from build123d import *

# Parameters (mm, degrees)
F2_W     = 2.1
F2_H     = 15
F2_W_2   = 15
F2_H_2   = 2.1
F2_R     = 1.5
F2_W_3   = 43.75
F2_H_3   = 19.25
F3_DEPTH = 1.5
F4_DEPTH = 4.7
F5_DEPTH = 6
F6_R     = 1.5


with BuildPart() as f3:
    # F2 (on Top) → F3 (new body)
    with BuildSketch(Plane.XY):
        Polygon((-51.25, 18.5100111359), (-51.25, 26.75), (-43.0100111359, 26.75), (-7.5, 26.75), (-7.5, 28.85), (-53.35, 28.85), (-53.35, 7.5), (-51.25, 7.5), align=None)
        with Locations((-52.3, 0)):
            Rectangle(F2_W, F2_H)
        with Locations((52.3, 0)):
            Rectangle(F2_W, F2_H)
        Polygon((7.5, 28.85), (7.5, 26.75), (43.0100111359, 26.75), (51.25, 26.75), (51.25, 18.5100111359), (51.25, 7.5), (53.35, 7.5), (53.35, 28.85), align=None)
        Polygon((-51.25, -18.5100111359), (-51.25, -7.5), (-53.35, -7.5), (-53.35, -28.85), (-7.5, -28.85), (-7.5, -26.75), (-43.0100111359, -26.75), (-51.25, -26.75), align=None)
        with Locations((0, -27.8)):
            Rectangle(F2_W_2, F2_H_2)
        with Locations((0, 27.8)):
            Rectangle(F2_W_2, F2_H_2)
        Polygon((53.35, -7.5), (51.25, -7.5), (51.25, -18.5100111359), (51.25, -26.75), (43.0100111359, -26.75), (7.5, -26.75), (7.5, -28.85), (53.35, -28.85), align=None)
        with BuildLine():
            Line((-7.5, -7.5), (-51.25, -7.5))
            Line((-51.25, -7.5), (-51.25, -18.5100111359))
            ThreePointArc((-51.25, -18.5100111359), (-43.3634253301, -18.8634253301), (-43.0100111359, -26.75))
            Line((-43.0100111359, -26.75), (-7.5, -26.75))
            Line((-7.5, -26.75), (-7.5, -7.5))
        make_face()
        with BuildLine():
            Line((-43.0100111359, 26.75), (-51.25, 26.75))
            Line((-51.25, 26.75), (-51.25, 18.5100111359))
            ThreePointArc((-51.25, 18.5100111359), (-43.3634253301, 18.8634253301), (-43.0100111359, 26.75))
        make_face()
        with Locations((-47.5, 23)):
            Circle(F2_R, mode=Mode.SUBTRACT)
        with BuildLine():
            Line((51.25, 26.75), (43.0100111359, 26.75))
            ThreePointArc((43.0100111359, 26.75), (43.3634253301, 18.8634253301), (51.25, 18.5100111359))
            Line((51.25, 18.5100111359), (51.25, 26.75))
        make_face()
        with Locations((47.5, 23)):
            Circle(F2_R, mode=Mode.SUBTRACT)
        with BuildLine():
            Line((51.25, -26.75), (51.25, -18.5100111359))
            ThreePointArc((51.25, -18.5100111359), (43.3634253301, -18.8634253301), (43.0100111359, -26.75))
            Line((43.0100111359, -26.75), (51.25, -26.75))
        make_face()
        with Locations((47.5, -23)):
            Circle(F2_R, mode=Mode.SUBTRACT)
        with BuildLine():
            ThreePointArc((-43.0100111359, -26.75), (-43.3634253301, -18.8634253301), (-51.25, -18.5100111359))
            Line((-51.25, -18.5100111359), (-51.25, -26.75))
            Line((-51.25, -26.75), (-43.0100111359, -26.75))
        make_face()
        with Locations((-47.5, -23)):
            Circle(F2_R, mode=Mode.SUBTRACT)
        with Locations((-29.375, 0)):
            Rectangle(F2_W_3, F2_H)
        with Locations((-47.5, 0)):
            Circle(F2_R, mode=Mode.SUBTRACT)
        with BuildLine():
            Line((-7.5, 26.75), (-43.0100111359, 26.75))
            ThreePointArc((-43.0100111359, 26.75), (-43.3634253301, 18.8634253301), (-51.25, 18.5100111359))
            Line((-51.25, 18.5100111359), (-51.25, 7.5))
            Line((-51.25, 7.5), (-7.5, 7.5))
            Line((-7.5, 7.5), (-7.5, 26.75))
        make_face()
        with Locations((0, 17.125)):
            Rectangle(F2_W_2, F2_H_3)
        with Locations((0, 23)):
            Circle(F2_R, mode=Mode.SUBTRACT)
        with BuildLine():
            Line((43.0100111359, 26.75), (7.5, 26.75))
            Line((7.5, 26.75), (7.5, 7.5))
            Line((7.5, 7.5), (51.25, 7.5))
            Line((51.25, 7.5), (51.25, 18.5100111359))
            ThreePointArc((51.25, 18.5100111359), (43.3634253301, 18.8634253301), (43.0100111359, 26.75))
        make_face()
        with Locations((29.375, 0)):
            Rectangle(F2_W_3, F2_H)
        with Locations((47.5, 0)):
            Circle(F2_R, mode=Mode.SUBTRACT)
        with BuildLine():
            Line((51.25, -7.5), (7.5, -7.5))
            Line((7.5, -7.5), (7.5, -26.75))
            Line((7.5, -26.75), (43.0100111359, -26.75))
            ThreePointArc((43.0100111359, -26.75), (43.3634253301, -18.8634253301), (51.25, -18.5100111359))
            Line((51.25, -18.5100111359), (51.25, -7.5))
        make_face()
        with Locations((0, -17.125)):
            Rectangle(F2_W_2, F2_H_3)
        with Locations((0, -23)):
            Circle(F2_R, mode=Mode.SUBTRACT)
        Rectangle(F2_W_2, F2_H)
    extrude(amount=F3_DEPTH)

    # F2 (on Top) → F4 (join)
    with BuildSketch(Plane.XY):
        with BuildLine():
            ThreePointArc((-43.0100111359, -26.75), (-43.3634253301, -18.8634253301), (-51.25, -18.5100111359))
            Line((-51.25, -18.5100111359), (-51.25, -26.75))
            Line((-51.25, -26.75), (-43.0100111359, -26.75))
        make_face()
        with Locations((-47.5, -23)):
            Circle(F2_R, mode=Mode.SUBTRACT)
        with BuildLine():
            Line((51.25, -26.75), (51.25, -18.5100111359))
            ThreePointArc((51.25, -18.5100111359), (43.3634253301, -18.8634253301), (43.0100111359, -26.75))
            Line((43.0100111359, -26.75), (51.25, -26.75))
        make_face()
        with Locations((47.5, -23)):
            Circle(F2_R, mode=Mode.SUBTRACT)
        with BuildLine():
            Line((51.25, 26.75), (43.0100111359, 26.75))
            ThreePointArc((43.0100111359, 26.75), (43.3634253301, 18.8634253301), (51.25, 18.5100111359))
            Line((51.25, 18.5100111359), (51.25, 26.75))
        make_face()
        with Locations((47.5, 23)):
            Circle(F2_R, mode=Mode.SUBTRACT)
        with BuildLine():
            Line((-43.0100111359, 26.75), (-51.25, 26.75))
            Line((-51.25, 26.75), (-51.25, 18.5100111359))
            ThreePointArc((-51.25, 18.5100111359), (-43.3634253301, 18.8634253301), (-43.0100111359, 26.75))
        make_face()
        with Locations((-47.5, 23)):
            Circle(F2_R, mode=Mode.SUBTRACT)
    extrude(amount=F4_DEPTH)

    # F2 (on Top) → F5 (join)
    with BuildSketch(Plane.XY):
        Polygon((-51.25, -18.5100111359), (-51.25, -7.5), (-53.35, -7.5), (-53.35, -28.85), (-7.5, -28.85), (-7.5, -26.75), (-43.0100111359, -26.75), (-51.25, -26.75), align=None)
        Polygon((53.35, -7.5), (51.25, -7.5), (51.25, -18.5100111359), (51.25, -26.75), (43.0100111359, -26.75), (7.5, -26.75), (7.5, -28.85), (53.35, -28.85), align=None)
        Polygon((-51.25, 18.5100111359), (-51.25, 26.75), (-43.0100111359, 26.75), (-7.5, 26.75), (-7.5, 28.85), (-53.35, 28.85), (-53.35, 7.5), (-51.25, 7.5), align=None)
        Polygon((7.5, 28.85), (7.5, 26.75), (43.0100111359, 26.75), (51.25, 26.75), (51.25, 18.5100111359), (51.25, 7.5), (53.35, 7.5), (53.35, 28.85), align=None)
    extrude(amount=F5_DEPTH)

    # F6
    f6_edges = [f3.edges().sort_by_distance(p)[0] for p in [
        (53.35, -28.85, 3),
        (53.35, 28.85, 3),
        (-53.35, 28.85, 3),
        (-53.35, -28.85, 3),
    ]]
    fillet(f6_edges, radius=F6_R)


solid = f3.part
Source: CAD feature listing. Evaluate the final solid. Frame: model axes, mm. A direction names the side the tool comes from. Round coordinates to 2 decimals unless told otherwise and drop trailing zeros. Loops run counter-clockwise (first coordinate to the right, second up) from the corner with the lowest first, then second, coordinate; pieces in that order, holes last. Notation, with made-up numbers: M -20.5,-15 L 20.5,-15 A12 ccw 20.5,-8 Z; hole C 72,31 d11. An arc over 180 degrees is marked long. Return JSON: item names as keys, results as strings. Group by question number.
1. Reachability of faces 1 (the face through (-52, -7.5, 4)), 2 (the face through (-49, -23, 2)), 3 (the face through (-7.5, 28, 4)), 4 (the face through (-47, -21, 4.7)) from +Z, -Z, +X, -X, +Y, -Y: full face, straight path, thin tool, end or side. Return the list, or none.
2. Pin query (flat end, axial travel): pin 1 (3.5 mm diameter, centred on x = -47.5, y = -23, fed in from -Z); pin 2 (0.6 mm diameter, centred on x = 53, z = 4, fed in from -Y); pin 3 (1.5 mm diameter, centred on x = -35, y = 2, fed in from +Z); pin 4 (1.8 mm diameter, centred on x = 47.5, y = -23, fed in from -Z). Return the tip coordinate at first contact, or that it passes through.
3. Section query C-C on y = 23. Output: boundary loops of the cut face in (x, z).
4. Mould query, pull axis Y, two halves, no side actions, for faces 5 (the face through (52, 7.5, 4)), 6 (the face through (35, -27, 6)). Classes: released by +Y, released by -Y, zero draft, split by the parting line, or undercut.
5. Section query B-B on x = 0. Output: boundary loops of the cut face in (y, z).
6. Section query D-D on x = -47.5. Output: boundary loops of the cut face in (y, z), and give its area (3 significant figures).
7. Section query A-A on y = 0. Output: boundary loops of the cut face in (x, z).
8. Material intervals for line 1 along Y through (x, z) = (47.5, 1); line 2 along Y through (x, z) = (30.5, 4.05); line 3 along Y through (x, z) = (0, 0.45), sorted ascending. Write a range as from..to.
Checks:
{
 "1": {"face 1": "+Z, +X, -X", "face 2": "+Z, -Z", "face 3": "+Z, +Y, -Y", "face 4": "+Z"},
 "2": {"pin 1": "stops at z = 0", "pin 2": "stops at y = -28.59", "pin 3": "stops at z = 1.5", "pin 4": "passes through"},
 "3": {"outline": "M -53.35,0 L -49,0 L -49,4.7 L -51.25,4.7 L -51.25,6 L -53.35,6 Z; M -46,0 L -1.5,0 L -1.5,1.5 L -41.65,1.5 L -41.65,4.7 L -46,4.7 Z; M 1.5,0 L 46,0 L 46,4.7 L 41.65,4.7 L 41.65,1.5 L 1.5,1.5 Z; M 49,0 L 53.35,0 L 53.35,6 L 51.25,6 L 51.25,4.7 L 49,4.7 Z"},
 "4": {"face 5": "undercut", "face 6": "zero draft"},
 "5": {"outline": "M -28.85,0 L -24.5,0 L -24.5,1.5 L -28.85,1.5 Z; M -21.5,0 L 21.5,0 L 21.5,1.5 L -21.5,1.5 Z; M 24.5,0 L 28.85,0 L 28.85,1.5 L 24.5,1.5 Z"},
 "6": {"outline": "M -28.85,0 L -24.5,0 L -24.5,4.7 L -26.75,4.7 L -26.75,6 L -28.85,6 Z; M -21.5,0 L -1.5,0 L -1.5,1.5 L -17.15,1.5 L -17.15,4.7 L -21.5,4.7 Z; M 1.5,0 L 21.5,0 L 21.5,4.7 L 17.15,4.7 L 17.15,1.5 L 1.5,1.5 Z; M 24.5,0 L 28.85,0 L 28.85,6 L 26.75,6 L 26.75,4.7 L 24.5,4.7 Z", "area": "134 mm²"},
 "7": {"outline": "M -53.35,0 L -49,0 L -49,1.5 L -53.35,1.5 Z; M -46,0 L 46,0 L 46,1.5 L -46,1.5 Z; M 49,0 L 53.35,0 L 53.35,1.5 L 49,1.5 Z"},
 "8": {"line 1": "y = -28.85..-24.5, -21.5..-1.5, 1.5..21.5, 24.5..28.85", "line 2": "y = -28.85..-26.75, 26.75..28.85", "line 3": "y = -28.85..-24.5, -21.5..21.5, 24.5..28.85"}
}
